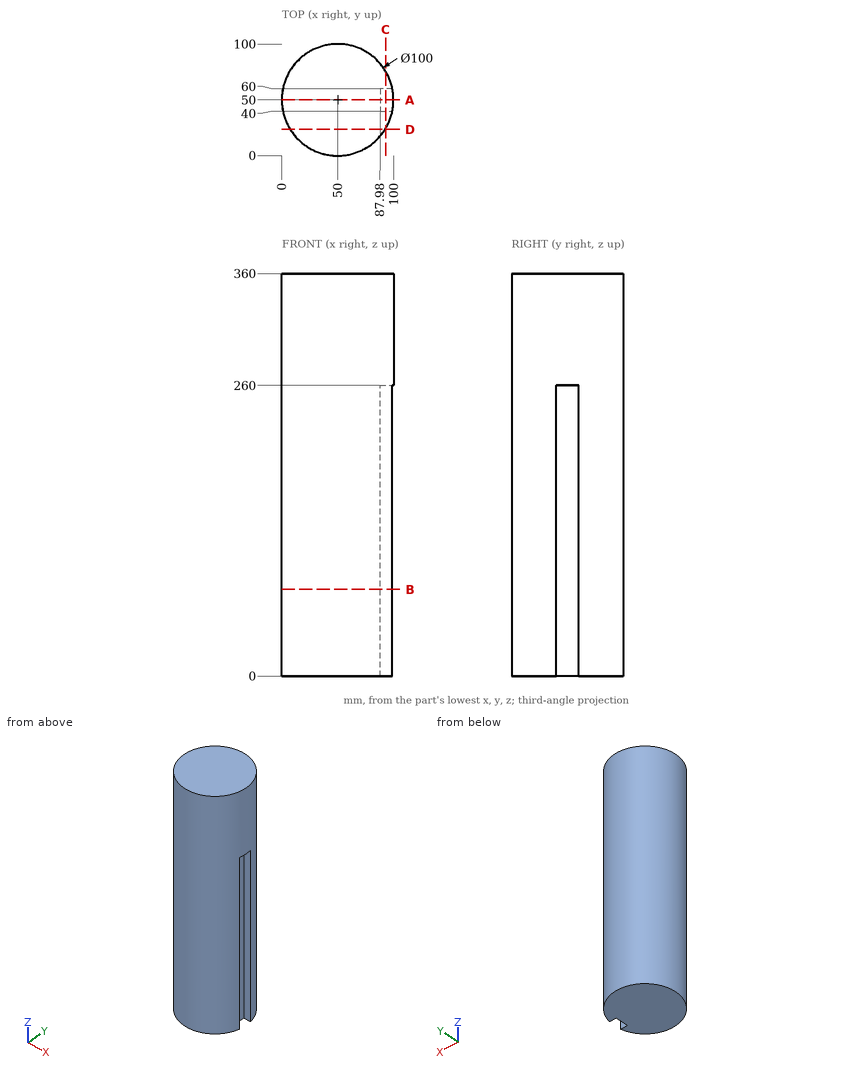
Input: dimensioned drawing with shaded views. Units: mm. Origin: part minimum x, y, z. Round coordinates to 2 decimals unless told otherwise and drop trailing zeros. Order: outer loops, then holes, each group sorted by start corner. A loop starts at its lowest first (then second) coordinate and runs counter-clockwise, first axis right, second up. Notation, with made-up numbers: (79.25, 68.25) -> (121.25, 68.25) arc R19 cw to (121.25, 86.25) -> close; hole circle Ø8 at (41, 82.5). An arc over 180 degrees is marked (long way). One line per item, written item: value. Start each with the question number.
Q1. Section query C-C (x = 93). Return the cut outline in (y, z) (1 decimal).
Q2. Pin query (flat end, axial travel): pin 1 (1.5 mm diameter, centred on x = 63.5, z = 146, fed in from +Y); pin 2 (16 mm diameter, centred on y = 45.5, z = 95, fed in from +X); pin 3 (12 mm diameter, centred on y = 21.5, z = 51.5, fed in from -X). Return the tip coordinate at first contact, or that it passes through.
Q3. Section query D-D (y = 23.5). Return the cut outline in (x, z), plus the area to 3 significant figures.
Q4. Material intervals for probe 1 along X at (y, z) = (48.5, 299.5); probe 2 along X at (y, z) = (52, 252); probe 3 along Y at (x, z) = (26, 209.5), sorted ascending.
Q5. Section query A-A (y = 50). Return the cut outline in (x, z), plus the area to 3 significant figures.
Q6. Section query B-B (z = 77.5). Return the cut outline in (x, y), plus the area to 3 significant figures.
Findings below:
1. outline: (24.5, 0) -> (40, 0) -> (40, 260) -> (60, 260) -> (60, 0) -> (75.5, 0) -> (75.5, 360) -> (24.5, 360) -> close
2. pin 1: y = 98.35
2. pin 2: x = 98.99
2. pin 3: x = 5.35
3. outline: (7.6, 0) -> (92.4, 0) -> (92.4, 360) -> (7.6, 360) -> close
3. area: 30,500 mm²
4. probe 1: 0.02 to 99.98
4. probe 2: 0.04 to 87.98
4. probe 3: 6.14 to 93.86
5. outline: (0, 0) -> (87.98, 0) -> (87.98, 260) -> (100, 260) -> (100, 360) -> (0, 360) -> close
5. area: 32,900 mm²
6. outline: (87.98, 40) -> (87.98, 60) -> (98.99, 60) arc R50 ccw (long way) to (98.99, 40) -> close
6. area: 7,620 mm²
